from build123d import *

# Parameters (mm, degrees)
SKETCH1_R           = 17
SKETCH1_R_2         = 1.8
SKETCH1_R_3         = 4.25
BOSS_EXTRUDE2_DEPTH = 3
BOSS_EXTRUDE4_START = -6
SKETCH2_R           = 1.8
BOSS_EXTRUDE4_DEPTH = 6
CIRPATTERN1_COUNT   = 8


with BuildPart() as part:
    # Sketch1 → Boss-Extrude2 (new body)
    with BuildSketch(Plane(origin=(0, 0, 0), x_dir=(1, 0, 0), z_dir=(0, 1, 0))):
        with Locations(Location((0, 0, 0), (0, 0, 270))):
            Circle(SKETCH1_R)
        with Locations(Location((-7.992388155, 9.192388155, 0), (0, 0, 270))):
            Circle(SKETCH1_R_2, mode=Mode.SUBTRACT)
        with Locations(Location((1.2, 0, 0), (0, 0, 270))):
            Circle(SKETCH1_R_3, mode=Mode.SUBTRACT)
        with Locations(Location((1.2, 13, 0), (0, 0, 270))):
            Circle(SKETCH1_R_2, mode=Mode.SUBTRACT)
        with Locations(Location((10.392388155, 9.192388155, 0), (0, 0, 270))):
            Circle(SKETCH1_R_2, mode=Mode.SUBTRACT)
        with Locations(Location((14.2, 0, 0), (0, 0, 270))):
            Circle(SKETCH1_R_2, mode=Mode.SUBTRACT)
        with Locations(Location((10.392388155, -9.192388155, 0), (0, 0, 270))):
            Circle(SKETCH1_R_2, mode=Mode.SUBTRACT)
        with Locations(Location((1.2, -13, 0), (0, 0, 270))):
            Circle(SKETCH1_R_2, mode=Mode.SUBTRACT)
        with Locations(Location((-7.992388155, -9.192388155, 0), (0, 0, 270))):
            Circle(SKETCH1_R_2, mode=Mode.SUBTRACT)
        with Locations(Location((-11.8, 0, 0), (0, 0, 270))):
            Circle(SKETCH1_R_2, mode=Mode.SUBTRACT)
    extrude(amount=BOSS_EXTRUDE2_DEPTH)

    # Sketch2 → Boss-Extrude4 (add)
    with BuildSketch(Plane(origin=(0, 3, 0), x_dir=(1, 0, 0), z_dir=(0, 1, 0)).offset(BOSS_EXTRUDE4_START)):
        with Locations(Location((-7.992388155, 9.192388155, 0), (0, 0, 270))):
            Circle(SKETCH2_R)
    boss_extrude4 = extrude(amount=BOSS_EXTRUDE4_DEPTH)

    # CirPattern1: Boss-Extrude4 ×8 about axis
    cirpattern1_axis = Axis((1.2, 0, 0), (0, 1, 0))
    for i in range(1, CIRPATTERN1_COUNT):
        add(boss_extrude4.rotate(cirpattern1_axis, i * 360 / CIRPATTERN1_COUNT))


solid = part.part
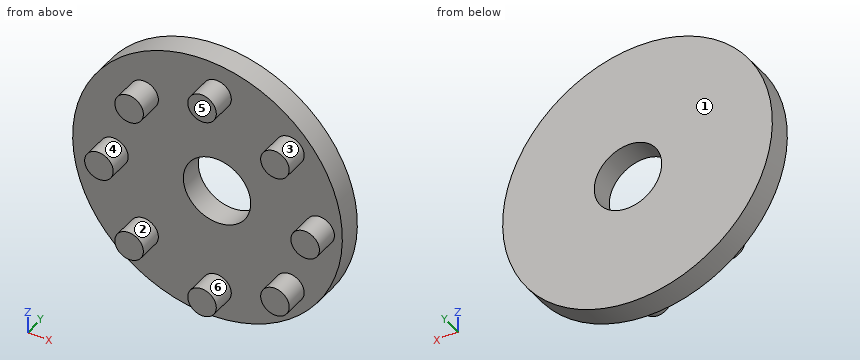
CAD build for the part. Positions are in the model's coordinates, mm. Face numbers are marked on the shaded views. A direction names the side the tool comes from. Round coordinates to 2 decimals unless told otherwise and drop trailing zeros. Order: outer loops, then holes, each group sorted by start corner. A loop starts at its lowest first (then second) coordinate and runs counter-clockwise, first axis right, second up. Notation, with made-up numbers: (-2, 71) - (40, 71) arc R15 ccw to (40, 80) - close; hole circle Ø5 at (1, 33.25). An arc over 180 degrees is marked (long way). Return JSON: item names as keys, results as strings.
(1) Wall check: probe 1 along X at (y, z) = (2, 0); probe 2 along Y at (x, z) = (1, 15.5); probe 3 along Z at (x, y) = (4.5, 2.6). Give the ranges that are in metal, low to high. Write a range as from..to.
Answer key:
{"probe 1": "x = -17..-3.05, 5.45..17", "probe 2": "y = 0..3", "probe 3": "z = -16.39..-2.68, 2.68..16.39"}
(2) Pin check, flat tips, straight feed: pin 1 Ø3 at (x, y) = (4.5, 1.5) entering from -Z; pin 2 Ø2 at (y, z) = (-2, -0.5) entering from +X; pin 3 Ø7 at (x, z) = (1.2, 0) entering from -Y; pin 4 Ø8 at (x, z) = (0, -3.5) entering from +Y. Stop position of each tip, or through.
Answer key:
{"pin 1": "stops at z = -16.73", "pin 2": "stops at x = 16", "pin 3": "passes through", "pin 4": "stops at y = 3"}
(3) Cut at B-B (x = 1.2). Give the cut face in (y, z), then the cut area to 3 significant figures.
Answer key:
{"outline": "(-3, -14.8) - (0, -14.8) - (0, -16.96) - (3, -16.96) - (3, -4.25) - (0, -4.25) - (0, -11.2) - (-3, -11.2) - close; (-3, 11.2) - (0, 11.2) - (0, 4.25) - (3, 4.25) - (3, 16.96) - (0, 16.96) - (0, 14.8) - (-3, 14.8) - close", "area": "97.8 mm^2"}
(4) Pull direction X, two halves, no side cores. Call the marked faces 3, 4, 5 and 6: +X half, -X half, draft (parallel to the pull), parting line (faces both ways), or undercut.
Answer key:
{"face 3": "undercut", "face 4": "undercut", "face 5": "draft", "face 6": "parting line"}
(5) Cut at C-C (y = 2.05). Give the cut face in (x, z).
Answer key:
{"outline": "circle Ø34 at (0, 0); hole circle Ø8.5 at (1.2, 0)"}
(6) Cut at A-A (z = 0). Give the cut face in (x, y), then the cut area to 3 significant figures.
Answer key:
{"outline": "(-17, 0) - (-13.6, 0) - (-13.6, -3) - (-10, -3) - (-10, 0) - (-3.05, 0) - (-3.05, 3) - (-17, 3) - close; (5.45, 0) - (12.4, 0) - (12.4, -3) - (16, -3) - (16, 0) - (17, 0) - (17, 3) - (5.45, 3) - close", "area": "98.1 mm^2"}
(7) Cut at D-D (x = 14.2). Give the cut face in (y, z).
Answer key:
{"outline": "(-3, -1.8) - (0, -1.8) - (0, -9.35) - (3, -9.35) - (3, 9.35) - (0, 9.35) - (0, 1.8) - (-3, 1.8) - close"}
(8) Tool access for the marked faces 1 and 2: list every direction of +Z, -Z, +X, -X, +Y, -Y with a clear straight run to the whole face (end or side of a thin tool).
Answer key:
{"face 1": "+Z, -Z, +X, -X, +Y", "face 2": "-Y"}
